Here's how the part is built. I have some questions about the finished solid (model axes, mm). A direction names the side the tool comes from. Round coordinates to 2 decimals unless told otherwise and drop trailing zeros. Order: outer loops, then holes, each group sorted by start corner. A loop starts at its lowest first (then second) coordinate and runs counter-clockwise, first axis right, second up. Notation, with made-up numbers: (54, -8) -> (83, -8) arc R21 ccw to (83, 21) -> close; hole circle Ø7 at (-27, -19.5). An arc over 180 degrees is marked (long way). One line per item, written item: value.
```python
from build123d import *

# Parameters (mm, degrees)
BOSS_EXTRUDE1_DEPTH = 3.175
SKETCH2_R           = 2.413
CUT_EXTRUDE1_DEPTH  = 146.311171514


with BuildPart() as part:
    # Sketch1 → Boss-Extrude1 (new body)
    with BuildSketch(Plane.XY):
        with BuildLine():
            Line((48.510867826, 121.831346212), (71.00638654, 30.794912365))
            ThreePointArc((71.00638654, 30.794912365), (70.423641708, 26.950767781), (67.293358183, 24.6446099))
            Line((67.293358183, 24.6446099), (54.964194654, 21.598017264))
            ThreePointArc((54.964194654, 21.598017264), (51.12005007, 22.180762096), (48.813892189, 25.311045622))
            Line((48.813892189, 25.311045622), (42.484535319, 50.925128378))
            ThreePointArc((42.484535319, 50.925128378), (40.684620517, 53.706308584), (37.552869907, 54.786491324))
            Line((37.552869907, 54.786491324), (2.614167294, 54.786491324))
            ThreePointArc((2.614167294, 54.786491324), (-0.977935154, 56.274388875), (-2.465832706, 59.866491324))
            Line((-2.465832706, 59.866491324), (-2.465832706, 120.308049894))
            ThreePointArc((-2.465832706, 120.308049894), (-0.605960766, 124.798177955), (3.884167294, 126.658049894))
            Line((3.884167294, 126.658049894), (42.346286061, 126.658049894))
            ThreePointArc((42.346286061, 126.658049894), (46.260974324, 125.30782147), (48.510867826, 121.831346212))
        make_face()
    extrude(amount=BOSS_EXTRUDE1_DEPTH)

    # Sketch2 → Cut-Extrude1 (cut, through all)
    with BuildSketch(Plane.XY.offset(3.175)):
        with Locations((58.082183783, 35.450477111)):
            Circle(SKETCH2_R)
        with Locations((48.942405878, 72.437967696)):
            Circle(SKETCH2_R)
        with Locations((39.802627972, 109.425458282)):
            Circle(SKETCH2_R)
        with Locations((10.234167294, 109.132049894)):
            Circle(SKETCH2_R)
        with Locations((10.234167294, 73.836491324)):
            Circle(SKETCH2_R)
    extrude(amount=-CUT_EXTRUDE1_DEPTH, mode=Mode.SUBTRACT)


solid = part.part
```
Q1. I want a section at C-C on x = 16. Write out the boundary of the cut face in (y, z) (1 decimal), then the cut area to 3 significant figures.
Answers:
outline: (54.8, 0) -> (126.7, 0) -> (126.7, 3.2) -> (54.8, 3.2) -> close
area: 228 mm2
Q2. I want a section at D-D on y = 80. Write out the boundary of the cut face in (x, z) (3 decimals).
Answers:
outline: (-2.466, 0) -> (58.848, 0) -> (58.848, 3.175) -> (-2.466, 3.175) -> close
Q3. I want a section at B-B on z = 0.65. Write out the boundary of the cut face in (x, y).
Answers:
outline: (-2.47, 59.87) arc R5.08 ccw to (2.61, 54.79) -> (37.55, 54.79) arc R5.08 cw to (42.48, 50.93) -> (48.81, 25.31) arc R5.08 ccw to (54.96, 21.6) -> (67.29, 24.64) arc R5.08 ccw to (71.01, 30.79) -> (48.51, 121.83) arc R6.35 ccw to (42.35, 126.66) -> (3.88, 126.66) arc R6.35 ccw to (-2.47, 120.31) -> close; hole circle Ø4.83 at (10.23, 73.84); hole circle Ø4.83 at (10.23, 109.13); hole circle Ø4.83 at (39.8, 109.43); hole circle Ø4.83 at (48.94, 72.44); hole circle Ø4.83 at (58.08, 35.45)
Q4. I need wall thicknesses on line 1 along Y through (x, z) = (7, 2.55); line 2 along X through (y, z) = (108, 2.8); line 3 along Y through (x, z) = (40.5, 2.3). Which ranges of each line are inside material? Lowest first, please.
Answers:
line 1: 54.79 to 126.66
line 2: -2.47 to 8.1, 12.37 to 37.86, 41.75 to 51.93
line 3: 53.84 to 107.12, 111.74 to 126.66
Q5. I want a section at A-A on x = 40. Write out the boundary of the cut face in (y, z) (3 decimals), then the cut area to 3 significant figures.
Answers:
outline: (54.158, 0) -> (107.021, 0) -> (107.021, 3.175) -> (54.158, 3.175) -> close; (111.83, 0) -> (126.658, 0) -> (126.658, 3.175) -> (111.83, 3.175) -> close
area: 215 mm2
Q6. Which directions (+Z, -Z, +X, -X, +Y, -Y) give clear straight access to the entire face, cutting with the end or side of a thin tool? Please do faces 1 (the face through (9.71, 71.48, 1.61)), 2 (the face through (20, 54.786, 2)).
Answers:
face 1: +Z, -Z
face 2: +Z, -Z, -X, -Y
Q7. If we mould it in two halves opening along Y, with no side actions, what happens to faces 3 (the face through (23, 126.658, 2)), 4 (the face through (45.694, 37.939, 1.565)), 5 (the face through (9.92, 111.525, 1.61))? For each: pulls with the +Y half, pulls with the -Y half, needs draft (parallel to the pull), parting line crosses it, or undercut.
Answers:
face 3: pulls with the +Y half
face 4: pulls with the -Y half
face 5: undercut
